Input: part model. Units: mm. Frame: model coordinates. Give positions to 0.01 mm unless a question says otherwise; leave off trailing zeros. Loops run counter-clockwise (first coordinate to the right, second up) from the corner with the lowest first, then second, coordinate; pieces in that order, holes last. Notation, with made-up numbers: M -33,47 L 8,47 A15 cw 8,70 Z; hole C 32,11 d6. An arc over 180 degrees is marked long. One line per item, written item: value. Start each with the question number.
(1) Section D-D on x = 27. Output: boundary loops of the cut face in (y, z).
(2) Section A-A on x = 56.5. Output: boundary loops of the cut face in (y, z).
(3) Pull-direction query (Z, two-part tool) for faces 1 (the flat face through (23, -2, 23)), 2 (the flat face through (57.7, -1, 30)); classes: released by +Z, released by -Z, zero draft, split by the parting line, or undercut.
(4) Section B-B on y = -1.4. State how many separate pieces and enclosed holes the cut face has, plus the area to 3 significant figures.
(5) Section C-C on z = 28. Output: boundary loops of the cut face in (x, y).
(6) Ray query, line 1 along X through (y, z) = (-1.35, 36); line 2 along X through (y, z) = (-0.45, 30.5). Return the intervals inside material, ascending. Write a range as from..to.
```python
from build123d import *

# Parameters (mm, degrees)
CROQUIS1_W              = 60.2
CROQUIS1_H              = 60.2
SALIENTE_EXTRUIR2_DEPTH = 2
CROQUIS1_5_W            = 14.8
CROQUIS1_5_H            = 2
CROQUIS1_5_W_2          = 2
CROQUIS1_5_H_2          = 14.8
CORTAR_EXTRUIR1_DEPTH   = 10


with BuildPart() as part:
    # Croquis1 → Saliente-Extruir2 (new body)
    with BuildSketch(Plane(origin=(0, 0, 0), x_dir=(1, 0, 0), z_dir=(0, 1, 0))):
        with Locations((30.1, -30.1)):
            Rectangle(CROQUIS1_W, CROQUIS1_H)
    extrude(amount=-SALIENTE_EXTRUIR2_DEPTH)

    # Croquis1_5 → Cortar-Extruir1 (cut)
    with BuildSketch(Plane(origin=(0, 0, 0), x_dir=(1, 0, 0), z_dir=(0, 1, 0))):
        with Locations((30.1, -56.7)):
            Rectangle(CROQUIS1_5_W, CROQUIS1_5_H)
        with Locations((30.1, -3.5)):
            Rectangle(CROQUIS1_5_W, CROQUIS1_5_H)
        with Locations((3.5, -30.1)):
            Rectangle(CROQUIS1_5_W_2, CROQUIS1_5_H_2)
        with Locations((56.7, -30.1)):
            Rectangle(CROQUIS1_5_W_2, CROQUIS1_5_H_2)
        Polygon((28.95, -22.7), (28.95, -28.95), (22.7, -28.95), (22.7, -31.25), (28.95, -31.25), (28.95, -37.5), (31.25, -37.5), (31.25, -31.25), (37.5, -31.25), (37.5, -28.95), (31.25, -28.95), (31.25, -22.7), align=None)
    extrude(amount=-CORTAR_EXTRUIR1_DEPTH, mode=Mode.SUBTRACT)


solid = part.part
```
Output values:
1. outline: M -2,0 L 0,0 L 0,2.5 L -2,2.5 Z; M -2,4.5 L 0,4.5 L 0,28.95 L -2,28.95 Z; M -2,31.25 L 0,31.25 L 0,55.7 L -2,55.7 Z; M -2,57.7 L 0,57.7 L 0,60.2 L -2,60.2 Z
2. outline: M -2,0 L 0,0 L 0,22.7 L -2,22.7 Z; M -2,37.5 L 0,37.5 L 0,60.2 L -2,60.2 Z
3. face 1: zero draft
3. face 2: undercut
4. separate pieces: 1
4. enclosed holes: 5
4. area: 3,440 mm²
5. outline: M 0,-2 L 2.5,-2 L 2.5,0 L 0,0 Z; M 4.5,-2 L 28.95,-2 L 28.95,0 L 4.5,0 Z; M 31.25,-2 L 55.7,-2 L 55.7,0 L 31.25,0 Z; M 57.7,-2 L 60.2,-2 L 60.2,0 L 57.7,0 Z
6. line 1: x = 0..2.5, 4.5..28.95, 31.25..55.7, 57.7..60.2
6. line 2: x = 0..2.5, 4.5..22.7, 37.5..55.7, 57.7..60.2
